Source: CAD feature listing. Evaluate the final solid. Frame: model axes, mm. Coordinates: 2 decimals unless noted, no trailing zeros. Order: outer loops, then holes, each group sorted by start corner. A loop starts at its lowest first (then second) coordinate and runs counter-clockwise, first axis right, second up.
Item 1: Section B-B on y = 12. Return the cut outline in (x, z) (3 decimals), then the cut area to 3 significant figures.
Item 2: Section C-C on z = 7.25. Return the cut outline in (x, y) (3 decimals), then the cut area to 3 significant figures.
Item 3: Contact query for a flat-ended pin moving along its axis: P1, Ø1, axis at y = 11, z = 8, coming from the -X side. Output: stop coordinate, or through.
Item 4: Section A-A on x = 35. Return the cut outline in (y, z) (3 decimals).
Item 5: Section D-D on x = 0. Return the cut outline in (y, z) (3 decimals).
Item 6: Ray query, line 1 (Y direction, x = 0, z = 7.5); line 2 (X direction, y = 4, z = 6.75); line 3 (X direction, y = 3, z = 8.5) (3 decimals). Return the intervals inside material, ascending.
Item 7: Mould query, pull axis Y, two halves, no side actions, for faces 1 (the cylindrical face through (-50.159, 6.178, 4.829)), 2 (the flat face through (53.975, 0, 5)), 3 (the cylindrical face through (20.52, 6.18, 4.83)), 4 (the cylindrical face through (49.43, -14.25, 4.83)). Classes: released by +Y, released by -Y, zero draft, split by the parting line, or undercut.
from build123d import *

# Parameters (mm, degrees)
F0_W     = 107.95
F0_H     = 38.1
F1_DEPTH = 9.525
F3_D     = 32.258
F5_D     = 32.258
F7_D     = 32.258
F8_R     = 15.943466
F9_R     = 15.9512
F10_R    = 15.9512
F11_R    = 15.9512


with BuildPart() as f1:
    # F0 (on Top) → F1 (new body)
    with BuildSketch(Plane.XY):
        Rectangle(F0_W, F0_H)
    extrude(amount=F1_DEPTH)

    # F3 (through all)
    with Locations(Plane.XY.offset(9.525)):
        with Locations((0, 0)):
            Hole(F3_D / 2)

    # F5 (through all)
    with Locations(Plane(origin=(0, 0, 0), x_dir=(1, 0, 0), z_dir=(0, 0, -1))):
        with Locations((-35.259712, 0)):
            Hole(F5_D / 2)

    # F7 (through all)
    with Locations(Plane(origin=(0, 0, 0), x_dir=(1, 0, 0), z_dir=(0, 0, -1))):
        with Locations((35.419382, 0)):
            Hole(F7_D / 2)

    # F8
    f8_edges = [f1.edges().sort_by_distance(p)[0] for p in [
        (53.975, 19.05, 4.7625),
    ]]
    fillet(f8_edges, radius=F8_R)

    # F9
    f9_edges = [f1.edges().sort_by_distance(p)[0] for p in [
        (53.975, -19.05, 4.7625),
    ]]
    fillet(f9_edges, radius=F9_R)

    # F10
    f10_edges = [f1.edges().sort_by_distance(p)[0] for p in [
        (-53.975, -19.05, 4.7625),
    ]]
    fillet(f10_edges, radius=F10_R)

    # F11
    f11_edges = [f1.edges().sort_by_distance(p)[0] for p in [
        (-53.975, 19.05, 4.7625),
    ]]
    fillet(f11_edges, radius=F11_R)


solid = f1.part
Answer list:
1. outline: (-51.26, 0) - (-46.037, 0) - (-46.037, 9.525) - (-51.26, 9.525) - close; (-24.483, 0) - (-10.777, 0) - (-10.777, 9.525) - (-24.483, 9.525) - close; (10.777, 0) - (24.642, 0) - (24.642, 9.525) - (10.777, 9.525) - close; (46.196, 0) - (51.264, 0) - (51.264, 9.525) - (46.196, 9.525) - close
1. area: 361 mm2
2. outline: (-53.975, -3.099) arc R15.951 ccw to (-38.024, -19.05) - (38.024, -19.05) arc R15.951 ccw to (53.975, -3.099) - (53.975, 3.107) arc R15.943 ccw to (38.032, 19.05) - (-38.024, 19.05) arc R15.951 ccw to (-53.975, 3.099) - close; hole circle Ø32.258 at (-35.26, 0); hole circle Ø32.258 at (0, 0); hole circle Ø32.258 at (35.419, 0)
2. area: 1,440 mm2
3. P1: stops at x = -52.15
4. outline: (-19.05, 0) - (-16.124, 0) - (-16.124, 9.525) - (-19.05, 9.525) - close; (16.124, 0) - (19.05, 0) - (19.05, 9.525) - (16.124, 9.525) - close
5. outline: (-19.05, 0) - (-16.129, 0) - (-16.129, 9.525) - (-19.05, 9.525) - close; (16.129, 0) - (19.05, 0) - (19.05, 9.525) - (16.129, 9.525) - close
6. line 1: y = -19.05 to -16.13, 16.13 to 19.05
6. line 2: x = -53.95 to -50.88, -19.63 to -15.63, 15.63 to 19.79, 51.04 to 53.95
6. line 3: x = -53.975 to -51.107, -19.412 to -15.848, 15.848 to 19.572, 51.267 to 53.975
7. face 1: undercut
7. face 2: zero draft
7. face 3: undercut
7. face 4: released by -Y
